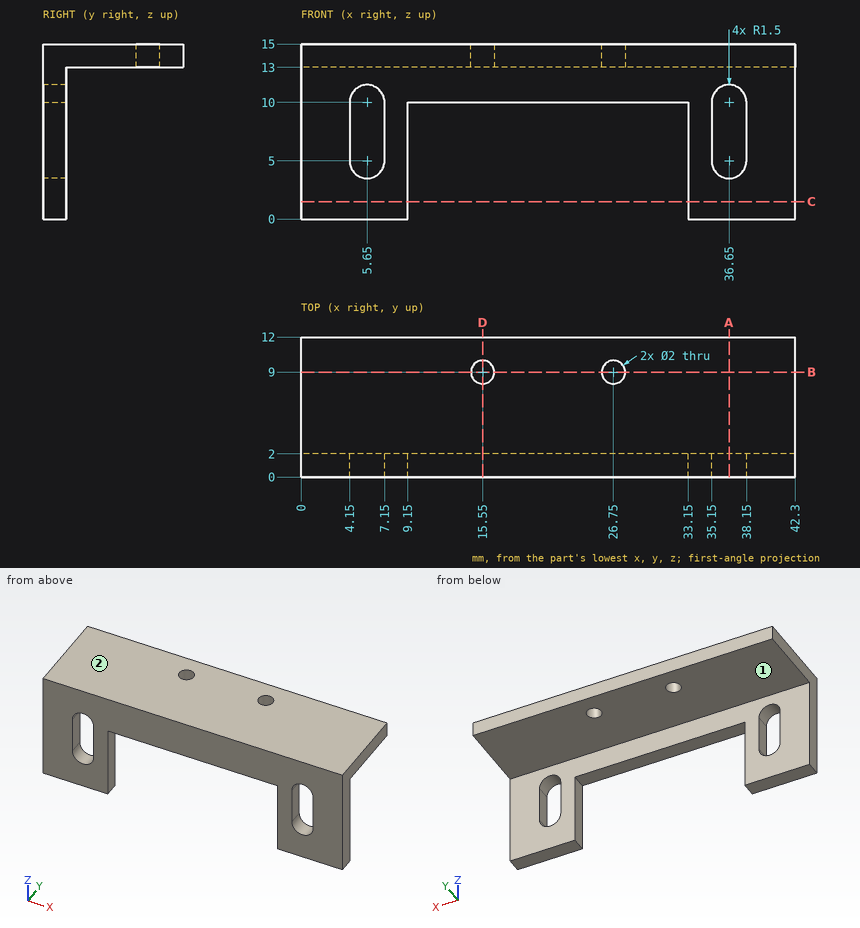
Input: dimensioned drawing with shaded views. Units: mm. Origin: part minimum x, y, z. A direction names the side the tool comes from. Coordinates: 2 decimals unless noted, no trailing zeros. Loops run counter-clockwise (first coordinate to the right, second up) from the corner with the lowest first, then second, coordinate; pieces in that order, holes last. Notation, with made-up numbers: M -26,-20 L 1,-20 A20 cw 1,-4 Z; hole C 87.5,-19.5 d6. An arc over 180 degrees is marked long. One line per item, written item: value.
(1) Line query: line 1 along Z through (x, y) = (21.5, 7); line 2 along Y through (x, z) = (26.75, 13.9); line 3 along Y through (x, z) = (15, 11.5). Output: solid intervals per line, ascending. Write a range as from..to.
Filled in:
line 1: 13..15
line 2: 0..8, 10..12
line 3: 0..2
(2) Section A-A (x = 36.65). Output: boundary loops of the cut face in (y, z).
Filled in:
outline: M 0,0 L 2,0 L 2,3.5 L 0,3.5 Z; M 0,11.5 L 2,11.5 L 2,13 L 12,13 L 12,15 L 0,15 Z
(3) Pin query (flat end, axial travel): pin 1 (5 mm diameter, centred on x = 21.5, y = 2.5, fed in from -Z); pin 2 (1.6 mm diameter, centred on y = 1, z = 7.5, fed in from -X). Return the tip coordinate at first contact, or that it passes through.
Filled in:
pin 1: z = 10
pin 2: x = 0
(4) Section B-B (y = 9). Output: boundary loops of the cut face in (x, z), and give its area (3 significant figures).
Filled in:
outline: M 0,13 L 14.55,13 L 14.55,15 L 0,15 Z; M 16.55,13 L 25.75,13 L 25.75,15 L 16.55,15 Z; M 27.75,13 L 42.3,13 L 42.3,15 L 27.75,15 Z
area: 76.6 mm^2
(5) Reachability of the marked faces 1 and 2 from +Z, -Z, +X, -X, +Y, -Y: full face, straight path, thin tool, end or side. Return the list, or none.
Filled in:
face 1: -Z, +X, -X, +Y
face 2: +Z, +X, -X, +Y, -Y
(6) Section D-D (x = 15.55). Output: boundary loops of the cut face in (y, z).
Filled in:
outline: M 0,10 L 2,10 L 2,13 L 8,13 L 8,15 L 0,15 Z; M 10,13 L 12,13 L 12,15 L 10,15 Z
(7) Section C-C (z = 1.5). Output: boundary loops of the cut face in (x, y).
Filled in:
outline: M 0,0 L 9.15,0 L 9.15,2 L 0,2 Z; M 33.15,0 L 42.3,0 L 42.3,2 L 33.15,2 Z
